Build history of the part. All positions in model axes, mm. Coordinates: 2 decimals unless noted, no trailing zeros. Order: outer loops, then holes, each group sorted by start corner. A loop starts at its lowest first (then second) coordinate and runs counter-clockwise, first axis right, second up. Notation, with made-up numbers: (36.5, 19.25) - (61.5, 19.25) arc R16 cw to (61.5, 49.25) - close; hole circle Ø5 at (68, -22.75). An arc over 180 degrees is marked (long way). One line per item, written item: value.
Autodesk Inventor part; units mm, degrees
ref_plane "Start Plane" through (0, 0, -6.1539) normal (0, 0, 1) x (1, 0, 0)
ref_plane "End Plane" through (0, 0, 175.0259) normal (0, 0, 1) x (1, 0, 0)
ref_plane "Work Plane4" through (-10.6086, -1.1246, -14.2686) normal (0.7964, 0.0844, -0.5988) x (-0.581, -0.1676, -0.7964)
ref_plane "Start Plane" through (0, 0, -6.1539) normal (0, 0, 1) x (1, 0, 0)
ref_plane "End Plane" through (0, 0, 175.0259) normal (0, 0, 1) x (1, 0, 0)
sketch "Sketch" plane through (0, 0, 0) normal (0, 0, 1) x (1, 0, 0)
  circle A0 centre (0, 0) radius 6.9342
  circle A1 centre (0, 0) radius 10.668
  dimension "d0" = 21.336
  dimension "d1" = 3.7338
extrude "Body" add sketch "Sketch" along normal up to surface (181.1798 mm away) from surface at -6.1539
sketch "Sketch3" plane through (0, 0, 0) normal (0, 0, 1) x (1, 0, 0)
  line L0 (0, 0) -> (10, 0)
ref_plane "Work Plane3" through (0, 0, 0) normal (0, -1, 0) x (1, 0, 0)
sketch "Sketch4" plane through (0, 0, 0) normal (0, -1, 0) x (1, 0, 0)
  line L0 (-2, -6.1539) -> (12, -6.1539)
  line L1 (-2, 175.0259) -> (12, 175.0259)
  dimension "d7" = 181.1798
ref_plane "Work Plane4" through (-10.6086, -1.1246, -14.2686) normal (0.7964, 0.0844, -0.5988) x (-0.581, -0.1676, -0.7964)
split "Split1" plane through (-10.6086, -1.1246, -14.2686) removes the side toward (0.7964, 0.0844, -0.5988)
ref_plane "Work Plane5" through (-2.0318, -10.4727, -6.2226) normal (0.096, 0.4946, -0.8638) x (0.9324, -0.3485, -0.096)
split "Split2" plane through (-2.0318, -10.4727, -6.2226) removes the side toward (0.096, 0.4946, -0.8638)
ref_plane "Work Plane6" through (8.2715, -6.7371, -19.1714) normal (-0.6775, 0.5518, -0.4862) x (0.1065, 0.7277, 0.6775)
split "Split3" plane through (8.2715, -6.7371, -19.1714) removes the side toward (-0.6775, 0.5518, -0.4862)
ref_plane "Work Plane7" through (-9.0832, -5.5948, 178.0591) normal (0.5074, 0.3125, 0.8031) x (0.8572, -0.0879, -0.5074)
split "Split4" plane through (-9.0832, -5.5948, 178.0591) removes the side toward (0.5074, 0.3125, 0.8031)
ref_plane "Work Plane8" through (-10.6086, -1.1246, 183.392) normal (0.7745, 0.0821, 0.6272) x (0.6313, -0.0391, -0.7745)
split "Split5" plane through (-10.6086, -1.1246, 183.392) removes the side toward (0.7745, 0.0821, 0.6272)
ref_plane "Work Plane9" through (6.6665, -8.3285, 178.5004) normal (-0.3854, 0.4815, 0.7872) x (0.9169, 0.1038, 0.3854)
split "Split6" plane through (6.6665, -8.3285, 178.5004) removes the side toward (-0.3854, 0.4815, 0.7872)
equation "\"d0\" = G_H"
equation "\"d1\" = G_T"
equation "\"d2\" = G_L"
equation "\"G_H\" = 21.336"
equation "\"G_T\" = 3.7338"
equation "\"G_L\" = 181.17984"
equation "\"G_OFFSET_START\" = 6.15394"
equation "\"G_OFFSET_END\" = 4.88279"
equation "\"d4\" = -G_OFFSET_START"
equation "\"d5\" = G_OFFSET_END + B_L"
equation "\"B_L\" = 170.14311"
properties part number "ANSI - 1/2 x 0.147 - 7.133" material "Steel, Mild"
1. Probe line 1 along Y through (x, z) = (0, 57.5); line 2 along Y through (x, z) = (5.5, 19). List the from-to ranges inside material, lowest first.
Values found:
line 1: y = -10.67 to -6.93, 6.93 to 10.67
line 2: y = -9.14 to -4.22, 4.22 to 9.14
2. Two-plate mould, pull along X, no slides. Class faces 1 (the face through (-7.25, 1.59, 11.91)), 2 (the face through (-1.389, -10.577, 83.168)), 3 (the face through (-0.903, -6.875, 83.417)), 4 (the face through (6.878, -2.883, 162.029)): pulls with the +X half, pulls with the -X half, needs draft (parallel to the pull), parting line crosses it, or undercut.
Values found:
face 1: pulls with the -X half
face 2: parting line crosses it
face 3: undercut
face 4: pulls with the +X half
3. Flat gauge pins, fed straight in: P1, Ø12, axis at x = 4, y = -7.5, coming from the -Z side; P2, Ø3, axis at y = 5, z = 70.5, coming from the +X side; P3, Ø10, axis at y = 6.5, z = 110, coming from the -X side. Where does each tip first touch, or does it go through?
Values found:
P1: stops at z = -3.76
P2: stops at x = 10.08
P3: stops at x = -10.56
4. Band-saw the part on B-B, the plane z = 94.5. Give the cut face in (x, y).
Values found:
outline: circle Ø21.34 at (0, 0); hole circle Ø13.87 at (0, 0)
5. Band-saw the part on C-C, the plane x = -8.5. Give the cut face in (y, z).
Values found:
outline: (-6.45, 4.53) - (6.45, 19.16) - (6.45, 162.04) - (-6.45, 169.92) - close
6. Band-saw the part on A-A, the plane y = 2. Give the cut face in (x, z).
Values found:
outline: (-10.48, 16.87) - (-6.64, 11.52) - (-6.64, 165.67) - (-10.48, 163.79) - close; (6.64, 9.11) - (10.48, 14.22) - (10.48, 156.94) - (6.64, 161.68) - close
